Geometry: final body of the model. Coordinates: model frame, mm. A direction names the side the tool comes from. Coordinates: 2 decimals unless noted, no trailing zeros. Loops run counter-clockwise (first coordinate to the right, second up) from the corner with the lowest first, then second, coordinate; pieces in that order, holes last. Notation, with made-up numbers: (74, 63.5) - (102, 63.5) arc R15 cw to (102, 89.5) - close; hole circle Ø2 at (-12.5, 49). An arc over 180 degrees is marked (long way). Put each result on its own line as item: value. Start each with the question number.
1) Reachability of faces 4 (the flat face through (15.293, 28.279, -634.435)), 5 (the flat face through (11.43, -3, -62)), 6 (the flat face through (9.39, 31.31, -765.79)), 7 (the flat face through (9.39, -177.07, -132.23)) from +Z, -Z, +X, -X, +Y, -Y: full face, straight path, thin tool, end or side. Return the list, or none.
2) Section C-C on y = 37. Output: boundary loops of the cut face in (x, z), and give its area (3 significant figures).
3) Material intervals for line 1 along Z through (x, y) = (12, 184.15); line 2 along Z through (x, y) = (16.75, 181); line 3 along Z through (x, y) = (14.5, -40.5), sorted ascending. Write a range as from..to.
4) Section B-B on y = 149. Output: boundary loops of the cut face in (x, z).
5) Contact query for flat-ended pins moving along their axis: pin 1 Ø6 at (x, z) = (16.5, -681.5) entering from +Y; pin 2 Ø9.5 at (y, z) = (-15.5, -64) entering from +X; pin 3 Ø1.5 at (x, z) = (12.5, -424) entering from +Y. Output: stop coordinate, or through.
6) Section A-A on x = 14.5. Count the separate pieces of the cut face and the enclosed holes in it, and give its area (3 significant figures).
7) Draft query along Z for faces 1 (the flat face through (9, 139, -811.342)), 2 (the flat face through (9.39, 175.73, -133.29)), 3 (the flat face through (9, 3, 77.658)). Return one class per face: +Z half, -Z half, draft (parallel to the pull), parting line (faces both ways), or undercut.
8) Section D-D on z = -299. Output: boundary loops of the cut face in (x, y), and give its area (3 significant figures).
```python
from build123d import *

# Parameters (mm, degrees)
F1_DEPTH = 19.05
F3_DEPTH = 7.62
F5_DEPTH = 7.62
F6_R     = 3.302
F6_R_2   = 5
F7_DEPTH = 19.05
F8_R     = 5
F9_DEPTH = 25.4


with BuildPart() as f1:
    # F0 (on Right) → F1 (new body)
    with BuildSketch(Plane.YZ):
        with BuildLine():
            Line((215.571838, -87.245801), (215.571838, 77.657629))
            Line((215.571838, 77.657629), (-216.228162, 77.657629))
            Line((-216.228162, 77.657629), (-216.228162, -87.245801))
            ThreePointArc((-216.228162, -87.245801), (-215.49657, -91.031394), (-213.407155, -94.271809))
            Line((-213.407155, -94.271809), (-139.7, -171.262371))
            Line((-139.7, -171.262371), (-139.7, -519.242371))
            Line((-139.7, -519.242371), (-215.9, -608.142371))
            Line((-215.9, -608.142371), (-215.9, -811.342371))
            Line((-215.9, -811.342371), (-63.5, -811.342371))
            Line((-63.5, -811.342371), (0, -721.487939))
            Line((0, -721.487939), (63.5, -811.342371))
            Line((63.5, -811.342371), (215.9, -811.342371))
            Line((215.9, -811.342371), (215.9, -741.492371))
            Line((215.9, -741.492371), (196.85, -741.492371))
            Line((196.85, -741.492371), (196.85, -639.892371))
            Line((196.85, -639.892371), (215.9, -639.892371))
            Line((215.9, -639.892371), (215.9, -608.142371))
            Line((215.9, -608.142371), (139.7, -519.242371))
            Line((139.7, -519.242371), (139.7, -171.262371))
            Line((139.7, -171.262371), (212.782136, -94.238963))
            ThreePointArc((212.782136, -94.238963), (214.848676, -91.010331), (215.571838, -87.245801))
        make_face()
    extrude(amount=F1_DEPTH)

    # F2 (on face) → F3 (cut)
    with BuildSketch(Plane.YZ.offset(19.05)):
        Polygon((191.608355, -700.919833), (196.842454, -682.602991), (-145.071934, -584.899811), (-150.306033, -603.216653), align=None)
    extrude(amount=-F3_DEPTH, mode=Mode.SUBTRACT)

    # F4 (on face) → F5 (cut)
    with BuildSketch(Plane.YZ.offset(19.05)):
        Polygon((-216.228162, -71.276438), (216.173725, -71.276438), (215.571838, -52.226438), (-216.228162, -52.226438), align=None)
    extrude(amount=-F5_DEPTH, mode=Mode.SUBTRACT)

    # F6 (on face) → F7 (cut)
    with BuildSketch(Plane.YZ):
        with Locations((-178.128162, -62.640438)):
            Circle(F6_R)
        with Locations((177.471838, -62.640438)):
            Circle(F6_R)
        with Locations((206.427838, 53.607629)):
            Circle(F6_R_2)
    extrude(amount=F7_DEPTH, mode=Mode.SUBTRACT)

    # F8 (on face) → F9 (cut)
    with BuildSketch(Plane.YZ):
        with Locations((184.15, -728.792371)):
            Circle(F8_R)
        with Locations((184.15, -652.592371)):
            Circle(F8_R)
    extrude(amount=F9_DEPTH, mode=Mode.SUBTRACT)


solid = f1.part
```
Answer block:
1. face 4: +X
1. face 5: +X, +Y, -Y
1. face 6: -Z, +X, -X
1. face 7: +X, -X, -Y
2. outline: (0, -773.84) - (19.05, -773.84) - (19.05, -656.74) - (11.43, -656.74) - (11.43, -636.93) - (19.05, -636.93) - (19.05, -71.28) - (11.43, -71.28) - (11.43, -52.23) - (19.05, -52.23) - (19.05, 77.66) - (0, 77.66) - close
2. area: 15,900 mm²
3. line 1: z = -811.34..-733.79, -723.79..-698.79, -678.98..-657.59, -647.59..-571.1, -124.42..-71.28, -52.23..77.66
3. line 2: z = -811.34..-732.68, -724.91..-697.89, -678.08..-656.48, -648.71..-567.43, -127.74..-71.28, -52.23..77.66
3. line 3: z = -778.8..-634.59, -614.78..-71.28, -52.23..77.66
4. outline: (0, -811.34) - (19.05, -811.34) - (19.05, -688.74) - (11.43, -688.74) - (11.43, -668.93) - (19.05, -668.93) - (19.05, -530.09) - (0, -530.09) - close; (0, -161.46) - (19.05, -161.46) - (19.05, -71.28) - (11.43, -71.28) - (11.43, -52.23) - (19.05, -52.23) - (19.05, 77.66) - (0, 77.66) - close
5. pin 1: stops at y = 196.85
5. pin 2: stops at x = 11.43
5. pin 3: stops at y = 139.7
6. separate pieces: 2
6. enclosed holes: 4
6. area: 295,000 mm²
7. face 1: -Z half
7. face 2: undercut
7. face 3: +Z half
8. outline: (0, -139.7) - (19.05, -139.7) - (19.05, 139.7) - (0, 139.7) - close
8. area: 5,320 mm²
